Geometry check sheet. Reference: the model listing, model coordinates, mm. Face numbers are marked on the shaded views. Give positions to 0.01 mm unless a question says otherwise; leave off trailing zeros. Loops run counter-clockwise (first coordinate to the right, second up) from the corner with the lowest first, then second, coordinate; pieces in that order, holes last. Notation, with made-up numbers: (-6.75, -9.75) - (23.25, -9.75) arc R21 cw to (23.25, 21.25) - close; hole circle Ø3 at (16.5, -17). An arc over 180 degrees is marked (long way). Write item = value, one per line. Start each with the question number.
from build123d import *

# Parameters (mm, degrees)
ESBO_O1_R                = 12.5
ESBO_O1_R_2              = 7.5
ESBO_O1_R_3              = 3
RESSALTO_EXTRUS_O2_DEPTH = 4.5


with BuildPart() as part:
    # Esboço1 → Ressalto-extrusão2 (new, symmetric)
    with BuildSketch(Plane.XY):
        with BuildLine():
            Line((-16.759819531, 89.565702497), (-54.759819531, -7.434297503))
            ThreePointArc((-54.759819531, -7.434297503), (-52.869139937, -24.144391432), (-38, -32))
            Line((-38, -32), (38, -32))
            ThreePointArc((38, -32), (52.869139937, -24.144391432), (54.759819531, -7.434297503))
            Line((54.759819531, -7.434297503), (16.759819531, 89.565702497))
            ThreePointArc((16.759819531, 89.565702497), (0, 101), (-16.759819531, 89.565702497))
        make_face()
        Circle(ESBO_O1_R, mode=Mode.SUBTRACT)
        with Locations((0, 83)):
            Circle(ESBO_O1_R_2, mode=Mode.SUBTRACT)
        with Locations((38, -14)):
            Circle(ESBO_O1_R_2, mode=Mode.SUBTRACT)
        with Locations((-38, -14)):
            Circle(ESBO_O1_R_2, mode=Mode.SUBTRACT)
        with Locations((0, -17.5)):
            Circle(ESBO_O1_R_3, mode=Mode.SUBTRACT)
        with Locations((15.155444566, 8.75)):
            Circle(ESBO_O1_R_3, mode=Mode.SUBTRACT)
        with Locations((-15.155444566, 8.75)):
            Circle(ESBO_O1_R_3, mode=Mode.SUBTRACT)
    extrude(amount=RESSALTO_EXTRUS_O2_DEPTH, both=True)


solid = part.part
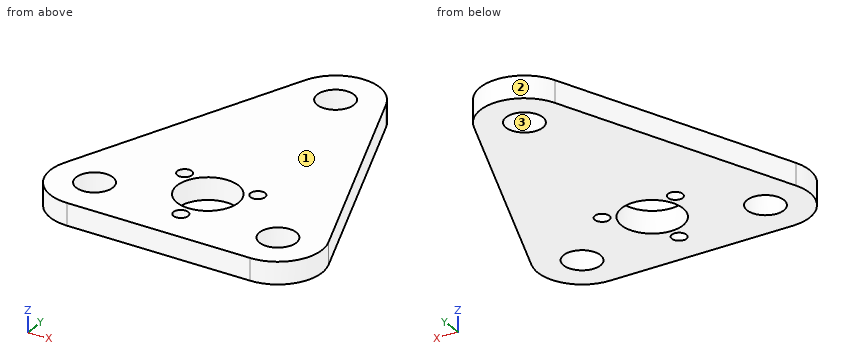
1) Cross-section at C-C on y = 88. Enter the section's corners in (x, z).
2) Material ranges on line 1 along Y through (x, z) = (0, -0.5); line 2 along X through (y, z) = (-16, -2); line 3 along Y through (x, z) = (-14, -2.5), recorded low to high.
3) Release check for a two-part mould opening along Y. For the marked faces 1, 2 and 3 record: pulls with the +Y half, pulls with the -Y half, needs draft (parallel to the pull), parting line crosses it, or undercut.
4) Cross-section at A-A on x = 0. Enter the section's corners in (y, z), and give its area (3 significant figures).
5) Gauge pin test, flat ends, axial feed: P1, Ø5, axis at x = 10, z = 1.5, coming from the +Y side; P2, Ø1.5, axis at y = -8, z = -2.5, coming from the -X side; P3, Ø17, axis at x = 0, y = 83, coming from the -Z side. Record the tip position at first contact, or that the pin passes through.
6) Cross-section at B-B on z = -0.75. Enter the section's corners in (x, y).
7) Cross-section at D-D on x = 14.5. Enter the section's corners in (y, z), and give its area (3 significant figures).
Checked values:
q1.outline = (-17.37, -4.5) - (-5.59, -4.5) - (-5.59, 4.5) - (-17.37, 4.5) - close; (5.59, -4.5) - (17.37, -4.5) - (17.37, 4.5) - (5.59, 4.5) - close
q2.line_1 = -32 to -20.5, -14.5 to -12.5, 12.5 to 75.5, 90.5 to 101
q2.line_2 = -55.89 to -45.23, -30.77 to -2.6, 2.6 to 30.77, 45.23 to 55.89
q2.line_3 = -32 to 5.98, 11.52 to 94.31
q3.face_1 = needs draft
q3.face_2 = pulls with the +Y half
q3.face_3 = undercut
q4.outline = (-32, -4.5) - (-20.5, -4.5) - (-20.5, 4.5) - (-32, 4.5) - close; (-14.5, -4.5) - (-12.5, -4.5) - (-12.5, 4.5) - (-14.5, 4.5) - close; (12.5, -4.5) - (75.5, -4.5) - (75.5, 4.5) - (12.5, 4.5) - close; (90.5, -4.5) - (101, -4.5) - (101, 4.5) - (90.5, 4.5) - close
q4.area = 783 mm²
q5.P1 = 99.36
q5.P2 = -55.22
q5.P3 = -4.5
q6.outline = (-54.76, -7.43) arc R18 ccw to (-38, -32) - (38, -32) arc R18 ccw to (54.76, -7.43) - (16.76, 89.57) arc R18 ccw to (-16.76, 89.57) - close; hole circle Ø15 at (-38, -14); hole circle Ø6 at (-15.16, 8.75); hole circle Ø25 at (0, 0); hole circle Ø15 at (0, 83); hole circle Ø6 at (0, -17.5); hole circle Ø6 at (15.16, 8.75); hole circle Ø15 at (38, -14)
q7.outline = (-32, -4.5) - (5.82, -4.5) - (5.82, 4.5) - (-32, 4.5) - close; (11.68, -4.5) - (93.67, -4.5) - (93.67, 4.5) - (11.68, 4.5) - close
q7.area = 1,080 mm²
